Print and shaded views of the part. All mm, measured from the part's lowest x, y and z. A direction names the side the tool comes from. Coordinates: 2 decimals unless noted, no trailing zeros. Order: outer loops, then holes, each group sorted by start corner. A loop starts at its lowest first (then second) coordinate and runs counter-clockwise, first axis right, second up. Notation, with made-up numbers: (35, -17.5) -> (39, -17.5) arc R24 ccw to (39, 14.5) -> close; hole circle Ø10 at (15, 66). An arc over 180 degrees is marked (long way). Return JSON: item names as keys, results as strings. Group by question number.
1) Probe line 1 (X direction, y = 15.25, z = 4.6); line 2 (X direction, y = 4, z = 0.7); line 3 (Y direction, x = 8.5, z = 2.9). List the from-to ranges inside material, lowest first.
2) Cut at B-B (y = 16.5). Write the cut outline in (x, z).
3) Which spindle directions (+Z, -Z, +X, -X, +Y, -Y) get a long thin tool onto all of the face, cutting with end or side? Do the marked faces 3, 4 and 5. Say none if no direction does.
4) Flat gauge pins, fed straight in: pin 1 (1.5 mm diameter, centred on x = 19, z = 4.5, fed in from -Y); pin 2 (3 mm diameter, centred on y = 3.5, z = 2, fed in from +X). Where does each tip first touch, or does it go through?
5) Pull direction X, two halves, no side cores. Call the marked faces 1 and 2: +X half, -X half, draft (parallel to the pull), parting line (faces both ways), or undercut.
6) Cut at C-C (z = 3.9). Write the cut outline in (x, y).
7) Cut at D-D (x = 54.5). Write the cut outline in (y, z).
8) Cut at A-A (y = 2). Write the cut outline in (x, z), and give its area (3 significant figures).
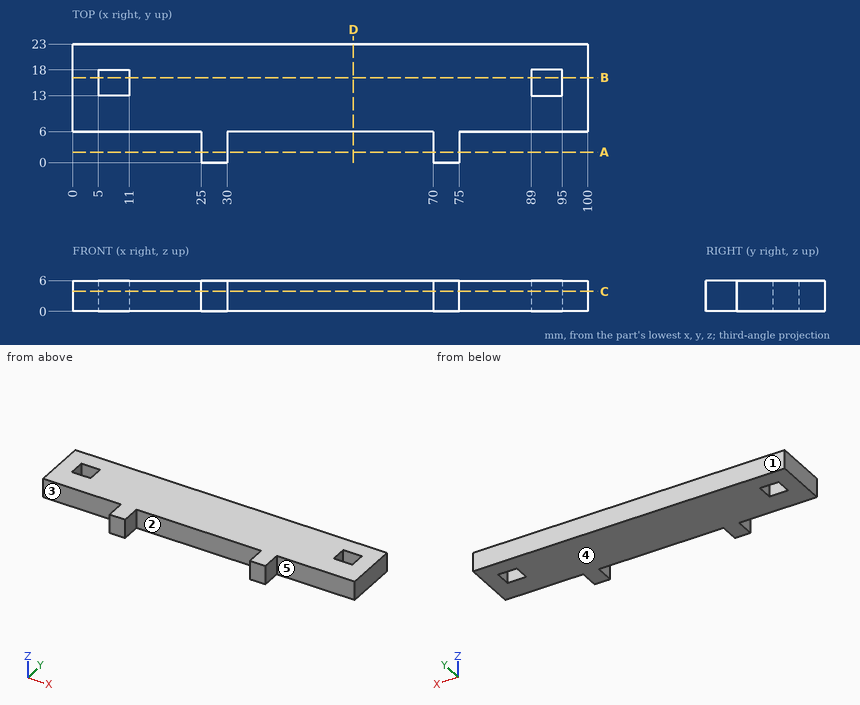
Answers below:
{
 "1": {"line 1": "x = 0 to 5, 11 to 89, 95 to 100", "line 2": "x = 25 to 30, 70 to 75", "line 3": "y = 6 to 13, 18 to 23"},
 "2": {"outline": "(0, 0) -> (5, 0) -> (5, 6) -> (0, 6) -> close; (11, 0) -> (89, 0) -> (89, 6) -> (11, 6) -> close; (95, 0) -> (100, 0) -> (100, 6) -> (95, 6) -> close"},
 "3": {"face 3": "+Z, -Z, -X, -Y", "face 4": "-Z, +X, -X, +Y, -Y", "face 5": "+Z, -Z, +X, -Y"},
 "4": {"pin 1": "stops at y = 6", "pin 2": "stops at x = 75"},
 "5": {"face 1": "draft", "face 2": "undercut"},
 "6": {"outline": "(0, 6) -> (25, 6) -> (25, 0) -> (30, 0) -> (30, 6) -> (70, 6) -> (70, 0) -> (75, 0) -> (75, 6) -> (100, 6) -> (100, 23) -> (0, 23) -> close; hole (5, 13) -> (11, 13) -> (11, 18) -> (5, 18) -> close; hole (89, 13) -> (95, 13) -> (95, 18) -> (89, 18) -> close"},
 "7": {"outline": "(6, 0) -> (23, 0) -> (23, 6) -> (6, 6) -> close"},
 "8": {"outline": "(25, 0) -> (30, 0) -> (30, 6) -> (25, 6) -> close; (70, 0) -> (75, 0) -> (75, 6) -> (70, 6) -> close", "area": "60.0 mm^2"}
}
